Can you work these out from the model? Positions are in its coordinate system, mm. A direction names the side the tool comes from. Give positions to 0.01 mm unless a question says otherwise; leave off trailing zeros. Write each loop counter-clockwise with the first axis right and the second up, starting at its lowest first coordinate (ties: lowest second). Pieces come first, ordered by that corner, then holes. Notation, with made-up numbers: (31, 64) -> (43, 64) arc R13 ccw to (43, 78) -> close; hole circle Ø6 at (30.25, 0). An arc over 180 degrees is marked (long way). Answer as CSV lines item,"result". Start each with the question number.
1. I'm going to push flat-ended pins straight in: P1, Ø1, axis at x = 1.5, z = 6.5, coming from the +Y side; P2, Ø2, axis at y = 0, z = 15.5, coming from the -X side; P3, Ø3, axis at x = 0, z = 14, coming from the +Y side. Where does each tip first touch, or does it pass through?
2. If we section it at B-B on x = 0: Write out the boundary of the cut face in (y, z), plus the area to 3 significant figures.
3. If we section it at D-D on x = -1: Write out the boundary of the cut face in (y, z), plus the area to 3 significant figures.
4. If we mould it in two halves opening along Z, with no side actions, what happens to faces 3 (the face through (3.233, -1.341, 0.986)), 4 (the face through (-0.028, 0.743, 14.689)), 5 (the face through (0, 0, 20))? For each: pulls with the +Z half, pulls with the -Z half, needs draft (parallel to the pull), parting line crosses it, or undercut.
5. I need wall thicknesses on line 1 (Z direction, x = 0.25, y = -3); line 2 (Y direction, x = 0.9, z = 15.5); line 3 (Z direction, x = 1.5, y = 1). Which ranges of each line are inside material? Lowest first, please. Write a range as [from, to].
6. If we section it at A-A on y = 0: Write out the boundary of the cut face in (x, z).
7. If we section it at C-C on z = 9.5: Write out the boundary of the cut face in (x, y).
8. On a 3-axis mill with a long thin cutter (end or side, diameter ignored), from which of +Z, -Z, +X, -X, +Y, -Y can I reach the whole of each face in a straight line? I mean faces 1 (the face through (0, 0, 0)), 2 (the face through (-2, 0, 11)). Say none if no direction works.
```python
from build123d import *

# Parameters (mm, degrees)
SZKIC1_R                    = 3.5
DODANIE_WYCI_GNI_CIE1_DEPTH = 2
SZKIC2_R                    = 2
DODANIE_WYCI_GNI_CIE2_DEPTH = 18
SZKIC3_R                    = 1.1
WYTNIJ_WYCI_GNI_CIE1_DEPTH  = 6.5


with BuildPart() as part:
    # Szkic1 → Dodanie-wyciągnięcie1 (new body)
    with BuildSketch(Plane.XY):
        Circle(SZKIC1_R)
    extrude(amount=DODANIE_WYCI_GNI_CIE1_DEPTH)

    # Szkic2 → Dodanie-wyciągnięcie2 (add)
    with BuildSketch(Plane.XY.offset(2)):
        Circle(SZKIC2_R)
    extrude(amount=DODANIE_WYCI_GNI_CIE2_DEPTH)

    # Szkic3 → Wytnij-wyciągnięcie1 (cut, through all)
    with BuildSketch(Plane.ZY.offset(2)):
        with Locations((15.5, 0)):
            Circle(SZKIC3_R)
    extrude(amount=-WYTNIJ_WYCI_GNI_CIE1_DEPTH, mode=Mode.SUBTRACT)


solid = part.part
```
Computed values:
1,P1,"stops at y = 1.73"
1,P2,"passes through"
1,P3,"stops at y = 2"
2,outline,"(-3.5, 0) -> (3.5, 0) -> (3.5, 2) -> (2, 2) -> (2, 20) -> (-2, 20) -> (-2, 2) -> (-3.5, 2) -> close; hole circle Ø2.2 at (0, 15.5)"
2,area,"82.2 mm2"
3,outline,"(-3.35, 0) -> (3.35, 0) -> (3.35, 2) -> (1.73, 2) -> (1.73, 20) -> (-1.73, 20) -> (-1.73, 2) -> (-3.35, 2) -> close; hole circle Ø2.2 at (0, 15.5)"
3,area,"72.0 mm2"
4,face 3,"needs draft"
4,face 4,"undercut"
4,face 5,"pulls with the +Z half"
5,line 1,"z = [0, 2]"
5,line 2,"y = [-1.79, -1.1], [1.1, 1.79]"
5,line 3,"z = [0, 15.04], [15.96, 20]"
6,outline,"(-3.5, 0) -> (3.5, 0) -> (3.5, 2) -> (2, 2) -> (2, 14.4) -> (-2, 14.4) -> (-2, 2) -> (-3.5, 2) -> close; (-2, 16.6) -> (2, 16.6) -> (2, 20) -> (-2, 20) -> close"
7,outline,"circle Ø4 at (0, 0)"
8,face 1,"-Z, +X, -X, +Y, -Y"
8,face 2,"+Z"
